from build123d import *

# Parameters (mm, degrees)
SKETCH_1_W          = 140
SKETCH_1_H          = 75
EXTRUDE_1_DEPTH     = 2
SKETCH_2_R          = 1.55
CUT_EXTRUDE_1_DEPTH = 3
SKETCH_3_W          = 7
SKETCH_3_H          = 55
EXTRUDE_2_DEPTH     = 62
SKETCH_5_R          = 1.55
CUT_EXTRUDE_2_DEPTH = 15
SKETCH_6_R          = 1.55
CUT_EXTRUDE_3_DEPTH = 15
SKETCH_7_W          = 4
SKETCH_7_H          = 52
CUT_EXTRUDE_4_DEPTH = 20


with BuildPart() as part:
    # 草图1 → 凸台-拉伸1 (new body)
    with BuildSketch(Plane(origin=(0, 0, 0), x_dir=(1, 0, 0), z_dir=(0, 1, 0))):
        Rectangle(SKETCH_1_W, SKETCH_1_H)
    extrude(amount=EXTRUDE_1_DEPTH)

    # 草图2 → 切除-拉伸1 (cut)
    with BuildSketch(Plane.XZ):
        with Locations(Location((-49, 0, 0), (0, 0, 270))):
            Circle(SKETCH_2_R)
        with Locations(Location((-49, -30, 0), (0, 0, 270))):
            Circle(SKETCH_2_R)
        with Locations(Location((-49, 30, 0), (0, 0, 270))):
            Circle(SKETCH_2_R)
        with Locations(Location((49, 30, 0), (0, 0, 270))):
            Circle(SKETCH_2_R)
        with Locations(Location((49, 0, 0), (0, 0, 270))):
            Circle(SKETCH_2_R)
        with Locations(Location((49, -30, 0), (0, 0, 270))):
            Circle(SKETCH_2_R)
    extrude(amount=-CUT_EXTRUDE_1_DEPTH, mode=Mode.SUBTRACT)

    # 草图3 → 凸台-拉伸2 (add)
    with BuildSketch(Plane.XZ):
        with Locations((-58.5, 0)):
            Rectangle(SKETCH_3_W, SKETCH_3_H)
        with Locations((58.5, 0)):
            Rectangle(SKETCH_3_W, SKETCH_3_H)
    extrude(amount=EXTRUDE_2_DEPTH)

    # 草图5 → 切除-拉伸2 (cut)
    with BuildSketch(Plane.XZ):
        with Locations(Location((-66, 20, 0), (0, 0, 270))):
            Circle(SKETCH_5_R)
        with Locations(Location((-66, 10, 0), (0, 0, 270))):
            Circle(SKETCH_5_R)
        with Locations(Location((-66, 0, 0), (0, 0, 270))):
            Circle(SKETCH_5_R)
        with Locations(Location((-66, -10, 0), (0, 0, 270))):
            Circle(SKETCH_5_R)
        with Locations(Location((-66, -20, 0), (0, 0, 270))):
            Circle(SKETCH_5_R)
        with Locations(Location((66, -20, 0), (0, 0, 270))):
            Circle(SKETCH_5_R)
        with Locations(Location((66, -10, 0), (0, 0, 270))):
            Circle(SKETCH_5_R)
        with Locations(Location((66, 0, 0), (0, 0, 270))):
            Circle(SKETCH_5_R)
        with Locations(Location((66, 10, 0), (0, 0, 270))):
            Circle(SKETCH_5_R)
        with Locations(Location((66, 20, 0), (0, 0, 270))):
            Circle(SKETCH_5_R)
    extrude(amount=-CUT_EXTRUDE_2_DEPTH, mode=Mode.SUBTRACT)

    # 草图6 → 切除-拉伸3 (cut)
    with BuildSketch(Plane.ZY.offset(62)):
        with Locations((-14.5, -54.5)):
            Circle(SKETCH_6_R)
        with Locations((14.5, -54.5)):
            Circle(SKETCH_6_R)
    cut_extrude_3 = extrude(amount=-CUT_EXTRUDE_3_DEPTH, mode=Mode.SUBTRACT)

    # 镜向1: 切除-拉伸3 across plane
    add(cut_extrude_3.mirror(Plane(origin=(0, 0, 0), x_dir=(0, 0, 1), z_dir=(1, 0, 0))), mode=Mode.SUBTRACT)

    # 草图7 → 切除-拉伸4 (cut)
    with BuildSketch(Plane.XZ.offset(62)):
        with Locations((58.5, 0)):
            Rectangle(SKETCH_7_W, SKETCH_7_H)
        with Locations((-58.5, 0)):
            Rectangle(SKETCH_7_W, SKETCH_7_H)
    extrude(amount=-CUT_EXTRUDE_4_DEPTH, mode=Mode.SUBTRACT)


solid = part.part
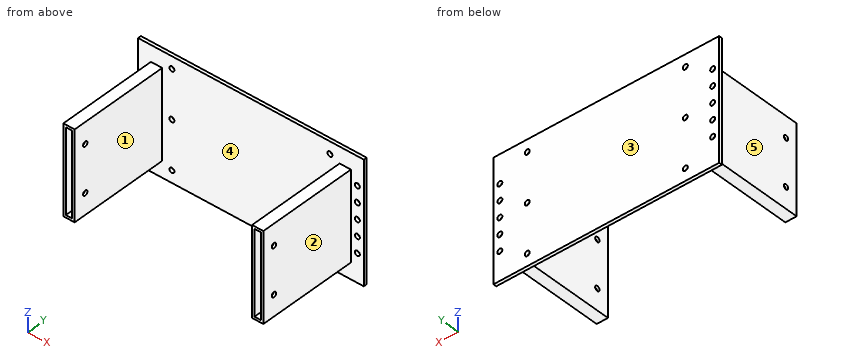
Input: part model. Units: mm. Frame: model coordinates. Face numbers are marked on the shaded views. A direction names the side the tool comes from. Give positions to 0.01 mm unless a question says otherwise; leave off trailing zeros. Write each loop counter-clockwise with the first axis right and the second up, starting at its lowest first coordinate (ties: lowest second). Pieces come first, ordered by that corner, then holes. Notation, with made-up numbers: M -38,82.5 L 21,82.5 A22 cw 21,96.5 Z; hole C 79,45 d2. An arc over 180 degrees is marked long. Write item = value, one per line. Start each with the question number.
1) Material intervals for line 1 along Z through (x, y) = (66, 0.9); line 2 along X through (y, z) = (-50, 3); line 3 along X through (y, z) = (1, -20), sorted ascending. Write a range as [from, to].
2) Cut plane D-D on x = 49. Return the cut outline in (y, z), then the cut area to 3 significant figures.
3) Cut plane A-A on z = -20. Return the cut outline in (x, y), then the cut area to 3 significant figures.
4) Cut plane C-C on y = -47. Return the cut outline in (x, z).
5) First-contact query: pin 1 Ø3 at (y, z) = (-54.5, -14.5) entering from +X; pin 2 Ø4 at (y, z) = (-34.5, 26.5) entering from +X; pin 3 Ø5 at (x, z) = (66, -10) entering from -Y; pin 4 Ø2 at (x, y) = (59.5, -50) entering from -Z. Flat tips, straight axial feed; report the tip coordinate or a pass-through.
6) Cut plane B-B on y = -25.5. Return the cut outline in (x, z), then the cut area to 3 significant figures.
7) Draft query along X for the marked faces 3, 4 and 5. Return one class per face: +X half, -X half, draft (parallel to the pull), parting line (faces both ways), or undercut.
8) Reachability of the marked faces 1 and 2 from +Z, -Z, +X, -X, +Y, -Y: full face, straight path, thin tool, end or side. Return the list, or none.
Solved:
q1.line_1 = [-37.5, -21.55], [-18.45, -11.55], [-8.45, -1.55], [1.55, 8.45], [11.55, 18.45], [21.55, 37.5]
q1.line_2 = [-62, -60.5], [-56.5, -55], [55, 56.5], [60.5, 62]
q1.line_3 = [-70, -67.55], [-64.45, 64.45], [67.55, 70]
q2.outline = M 0,-37.5 L 2,-37.5 L 2,-31.55 L 0,-31.55 Z; M 0,-28.45 L 2,-28.45 L 2,-1.55 L 0,-1.55 Z; M 0,1.55 L 2,1.55 L 2,28.45 L 0,28.45 Z; M 0,31.55 L 2,31.55 L 2,37.5 L 0,37.5 Z
q2.area = 131 mm2
q3.outline = M -70,0 L -67.55,0 L -67.55,2 L -70,2 Z; M -64.45,0 L -62,0 L -62,-62 L -60.5,-62 L -60.5,-42 L -56.5,-42 L -56.5,-62 L -55,-62 L -55,0 L 55,0 L 55,-62 L 56.5,-62 L 56.5,-42 L 60.5,-42 L 60.5,-62 L 62,-62 L 62,0 L 64.45,0 L 64.45,2 L -64.45,2 Z; M 67.55,0 L 70,0 L 70,2 L 67.55,2 Z
q3.area = 976 mm2
q4.outline = M -62,-27.5 L -55,-27.5 L -55,27.5 L -62,27.5 Z; M 55,-27.5 L 62,-27.5 L 62,27.5 L 55,27.5 Z; hole M -60.5,-26 L -56.5,-26 L -56.5,26 L -60.5,26 Z; hole M 56.5,-26 L 60.5,-26 L 60.5,26 L 56.5,26 Z
q5.pin_1 = through
q5.pin_2 = 62
q5.pin_3 = 0
q5.pin_4 = -27.5
q6.outline = M -62,-27.5 L -55,-27.5 L -55,27.5 L -62,27.5 Z; M 55,-27.5 L 62,-27.5 L 62,27.5 L 55,27.5 Z
q6.area = 770 mm2
q7.face_3 = draft
q7.face_4 = undercut
q7.face_5 = -X half
q8.face_1 = +Z, -Z, -Y
q8.face_2 = +Z, -Z, +X, -Y
